Can you work these out from the model? Positions are in its coordinate system, mm. Give positions to 0.01 mm unless a question says otherwise; leave off trailing zeros. Loops run counter-clockwise (first coordinate to the right, second up) from the corner with the lowest first, then second, coordinate; pieces in that order, holes last. Notation, with made-up numbers: (-34.75, -36) -> (-14.75, -36) arc R16 cw to (-14.75, -23) -> close; hole circle Ø10 at (-33, -9.5). An arc over 180 degrees is marked (long way). Return JSON: item names as keys, results as strings. Group by question number.
Q1. Suppose I cut it at C-C, the plane x = 582. Please give me the cut outline in (y, z).
Q2. Will these pins go through, and if not, where does the flat tip stop? pin 1 (2 mm diameter, centred on y = 111, z = 7.5, fed in from +X); pin 2 (5 mm diameter, centred on y = 110.5, z = 1, fed in from +X); pin 3 (6 mm diameter, centred on y = 79, z = 2.5, fed in from +X).
Q3. I need wall thicknesses on line 1 along Y through (x, z) = (346.5, 3); line 2 along X through (y, z) = (-10, 4); line 3 along X through (y, z) = (-93.5, 9.5). Which ranges of each line are inside material? Lowest first, please. Write a range as [from, to].
Q4. Suppose I cut it at A-A, the plane z = 5.75. Please give me the cut outline in (x, y), and give its area (3 significant figures).
Q5. Suppose I cut it at B-B, the plane x = 101. Please give me the cut outline in (y, z), and give its area (3 significant figures).
```python
from build123d import *

# Parameters (mm, degrees)
F2_DEPTH = 10
F4_DEPTH = 10.001
F6_DEPTH = 2


with BuildPart() as f2:
    # F1 (on Top) → F2 (new body)
    with BuildSketch(Plane.XY):
        with BuildLine():
            Line((375, 125), (0, 125))
            Line((0, 125), (-375, 125))
            Line((-375, 125), (-750, 175))
            ThreePointArc((-750, 175), (-949.8820360883, 0), (-750, -175))
            Line((-750, -175), (-375, -125))
            Line((-375, -125), (0, -125))
            Line((0, -125), (375, -125))
            Line((375, -125), (750, -175))
            ThreePointArc((750, -175), (949.8820360883, 0), (750, 175))
            Line((750, 175), (375, 125))
        make_face()
    extrude(amount=F2_DEPTH)

    # F3 (on face) → F4 (cut, through all)
    with BuildSketch(Plane.XY.offset(10)):
        with BuildLine():
            Line((-543, -147.4), (-475, -138.3333333333))
            Line((-475, -138.3333333333), (-480.5508762438, -96.7017615047))
            ThreePointArc((-480.5508762438, -96.7017615047), (-516.1668220423, -89.1155013498), (-548.5508762438, -105.7684281713))
            Line((-548.5508762438, -105.7684281713), (-543, -147.4))
        make_face()
    extrude(amount=-F4_DEPTH, mode=Mode.SUBTRACT)

    # F5 (on face) → F6 (cut)
    with BuildSketch(Plane(origin=(0, 0, 0), x_dir=(1, 0, 0), z_dir=(0, 0, -1))):
        with BuildLine():
            Line((-543, 147.4), (-574, 151.5333333333))
            Line((-574, 151.5333333333), (-576.6432744018, 131.7087753197))
            ThreePointArc((-576.6432744018, 131.7087753197), (-520.3099410685, 58.042108653), (-446.6432744018, 114.3754419863))
            Line((-446.6432744018, 114.3754419863), (-444, 134.2))
            Line((-444, 134.2), (-475, 138.3333333333))
            Line((-475, 138.3333333333), (-480.5508762438, 96.7017615047))
            ThreePointArc((-480.5508762438, 96.7017615047), (-516.1668220423, 89.1155013498), (-548.5508762438, 105.7684281713))
            Line((-548.5508762438, 105.7684281713), (-543, 147.4))
        make_face()
    extrude(amount=-F6_DEPTH, mode=Mode.SUBTRACT)


solid = f2.part
```
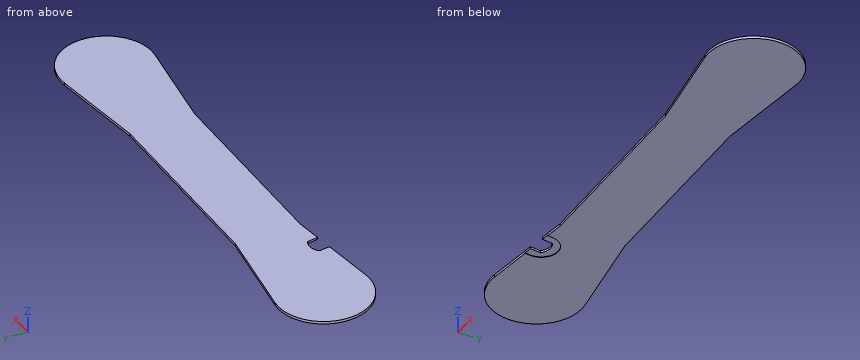
Ans:
{
 "1": {"outline": "(-152.6, 0) -> (152.6, 0) -> (152.6, 10) -> (-152.6, 10) -> close"},
 "2": {"pin 1": "stops at x = 911.43", "pin 2": "stops at x = 913", "pin 3": "stops at x = 932.69"},
 "3": {"line 1": "y = [-125, 125]", "line 2": "x = [-949.6, 949.6]", "line 3": "x = [-923.09, -531.44], [-486.56, 923.09]"},
 "4": {"outline": "(-750, -175) -> (-543, -147.4) -> (-548.55, -105.77) arc R54.23 cw to (-480.55, -96.7) -> (-475, -138.33) -> (-375, -125) -> (375, -125) -> (750, -175) arc R176.55 ccw (long way) to (750, 175) -> (375, 125) -> (-375, 125) -> (-750, 175) arc R176.55 ccw (long way) to start", "area": "523,000 mm^2"},
 "5": {"outline": "(-125, 0) -> (125, 0) -> (125, 10) -> (-125, 10) -> close", "area": "2,500 mm^2"}
}
